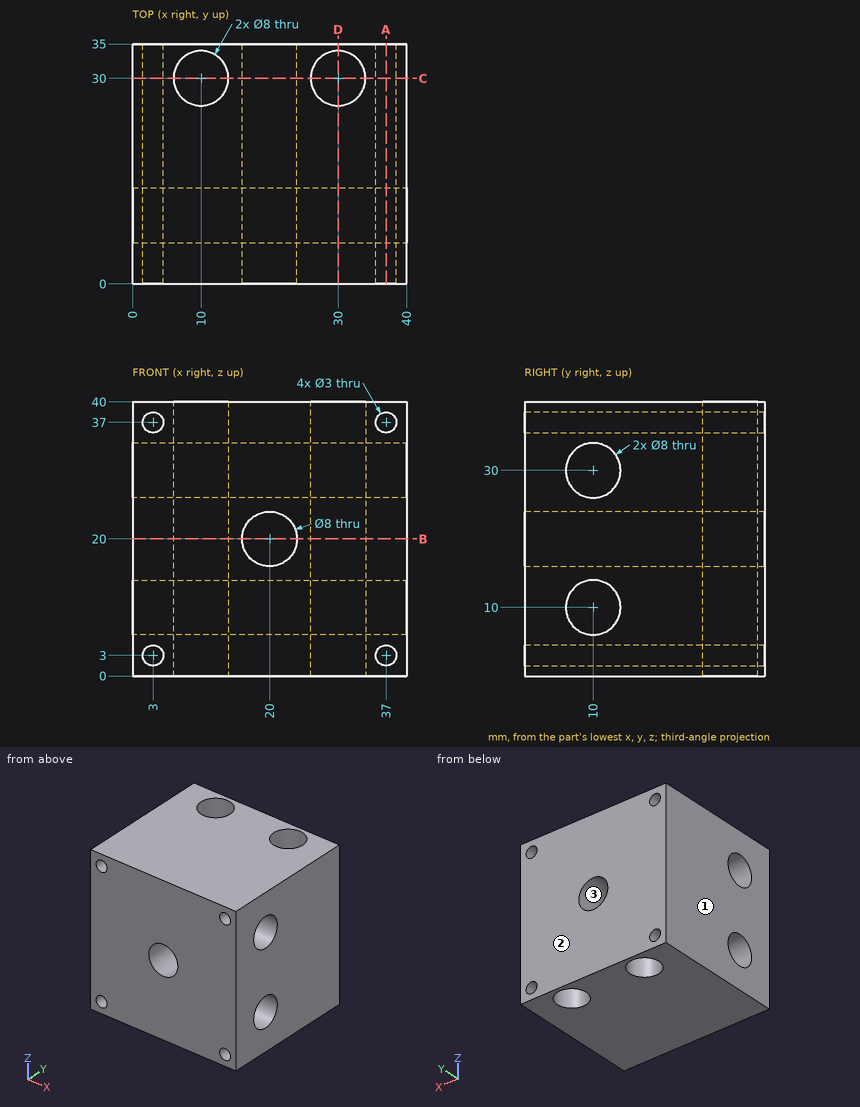
Geometry check sheet. Reference: drawing and pictorial views, mm from the part's lowest x, y, z. Round coordinates to 2 decimals unless told otherwise and drop trailing zeros. Write each loop counter-clockwise with the first axis right and the second up, starting at its lowest first coordinate (ties: lowest second). Pieces come first, ordered by that corner, then holes. Notation, with made-up numbers: (62, 40) -> (97, 40) arc R32 ccw to (97, 74) -> close; hole circle Ø10 at (45.25, -36.75). An arc over 180 degrees is marked (long way). Answer as CSV lines item,"result". Start each with the question number.
1) Section check C-C on y = 30. Enter the section's corners in (x, z), and give its area (3 significant figures).
2) Release check for a two-part mould opening along X. For the marked faces 1, 2 and 3 record: pulls with the +X half, pulls with the -X half, needs draft (parallel to the pull), parting line crosses it, or undercut.
3) Section check B-B on z = 20. Enter the section's corners in (x, y), and give its area (3 significant figures).
4) Material ranges on line 1 (X direction, y = 21, z = 3); line 2 (Z direction, x = 36.5, y = 9.5); line 3 (Z direction, x = 22, y = 10.5), recorded low to high. Write a range as from..to.
5) Section check D-D on x = 30. Enter the section's corners in (y, z).
6) Go/stop test with flat-tipped pins: P1, Ø2, axis at y = 14, z = 7.5, coming from the -X side; P2, Ø6.5, axis at y = 10, z = 30, coming from the +X side. Record where each tip stops, or that it passes through.
7) Section check A-A on x = 37. Enter the section's corners in (y, z).
Found:
1,outline,"(0, 0) -> (6, 0) -> (6, 40) -> (0, 40) -> close; (14, 0) -> (26, 0) -> (26, 40) -> (14, 40) -> close; (34, 0) -> (40, 0) -> (40, 40) -> (34, 40) -> close; hole circle Ø3 at (3, 3); hole circle Ø3 at (3, 37); hole circle Ø8 at (20, 20); hole circle Ø3 at (37, 3); hole circle Ø3 at (37, 37)"
1,area,"881 mm^2"
2,face 1,"pulls with the -X half"
2,face 2,"needs draft"
2,face 3,"undercut"
3,outline,"(0, 0) -> (16, 0) -> (16, 35) -> (0, 35) -> close; (24, 0) -> (40, 0) -> (40, 35) -> (24, 35) -> close; hole circle Ø8 at (10, 30); hole circle Ø8 at (30, 30)"
3,area,"1,020 mm^2"
4,line 1,"x = 0..1.5, 4.5..35.5, 38.5..40"
4,line 2,"z = 0..1.59, 4.41..6.03, 13.97..26.03, 33.97..35.59, 38.41..40"
4,line 3,"z = 0..6.03, 13.97..16.54, 23.46..26.03, 33.97..40"
5,outline,"(0, 0) -> (26, 0) -> (26, 40) -> (0, 40) -> close; (34, 0) -> (35, 0) -> (35, 40) -> (34, 40) -> close; hole circle Ø8 at (10, 10); hole circle Ø8 at (10, 30)"
6,P1,"stops at x = 0"
6,P2,"passes through"
7,outline,"(0, 0) -> (35, 0) -> (35, 1.5) -> (0, 1.5) -> close; (0, 4.5) -> (35, 4.5) -> (35, 35.5) -> (0, 35.5) -> close; (0, 38.5) -> (35, 38.5) -> (35, 40) -> (0, 40) -> close; hole circle Ø8 at (10, 10); hole circle Ø8 at (10, 30)"
